Build history of the part. All positions in model axes, mm. Face numbers are marked on the shaded views. Give positions to 0.01 mm unless a question says otherwise; leave off trailing zeros. Order: outer loops, then holes, each group sorted by start corner. A loop starts at its lowest first (then second) coordinate and runs counter-clockwise, first axis right, second up. Notation, with made-up numbers: (-30.75, -37) - (18.25, -37) arc R13 ccw to (18.25, -32) - close; hole circle Ø3 at (71.5, -24.75). An arc over 180 degrees is marked (long way). Use a Markdown table: item, result.
from build123d import *

# Parameters (mm, degrees)
SKETCH1_R           = 2.5
BOSS_EXTRUDE1_DEPTH = 20
CHAMFER1_SIZE       = 0.1
CHAMFER1_SIZE2      = 0.235585237
CUT_EXTRUDE1_DEPTH  = 0.5
FILLET1_R           = 0.05


with BuildPart() as part:
    # Sketch1 → Boss-Extrude1 (new body)
    with BuildSketch(Plane(origin=(0, 0, 0), x_dir=(1, 0, 0), z_dir=(0, 1, 0))):
        with Locations(Location((0, 0, 0), (0, 0, 270))):
            Circle(SKETCH1_R)
    extrude(amount=BOSS_EXTRUDE1_DEPTH)

    # Chamfer1
    chamfer1_edges = [part.edges().sort_by_distance(p)[0] for p in [
        (0, 20, -2.5),
    ]]
    chamfer1_side = [part.faces().sort_by_distance(p)[0] for p in [
        (0, 10, -2.5),
    ]]
    chamfer(chamfer1_edges, length=CHAMFER1_SIZE, length2=CHAMFER1_SIZE2, reference=chamfer1_side[0])

    # Sketch2 → Cut-Extrude1 (cut)
    with BuildSketch(Plane(origin=(0, 20, 0), x_dir=(1, 0, 0), z_dir=(0, 1, 0))):
        Polygon((0.5, 0.5), (0.5, 1.5), (-0.5, 1.5), (-0.5, 0.5), (-1.5, 0.5), (-1.5, -0.5), (-0.5, -0.5), (-0.5, -1.5), (0.5, -1.5), (0.5, -0.5), (1.5, -0.5), (1.5, 0.5), align=None)
    extrude(amount=-CUT_EXTRUDE1_DEPTH, mode=Mode.SUBTRACT)

    # Fillet1
    fillet1_edges = [part.edges().sort_by_distance(p)[0] for p in [
        (-0.5, 19.5, -1),
        (0, 19.5, -1.5),
        (0.5, 19.5, -1),
        (1, 19.5, -0.5),
        (1.5, 19.5, 0),
        (1, 19.5, 0.5),
        (0.5, 19.5, 1),
        (0, 19.5, 1.5),
        (-0.5, 19.5, 1),
        (-1, 19.5, 0.5),
        (-1.5, 19.5, 0),
        (-1, 19.5, -0.5),
        (-0.5, 20, -1),
        (-1, 20, -0.5),
        (-1.5, 20, 0),
        (-1, 20, 0.5),
        (-0.5, 20, 1),
        (0, 20, 1.5),
        (0.5, 20, 1),
        (1, 20, 0.5),
        (1.5, 20, 0),
        (1, 20, -0.5),
        (0.5, 20, -1),
        (0, 20, -1.5),
    ]]
    fillet(fillet1_edges, radius=FILLET1_R)


solid = part.part
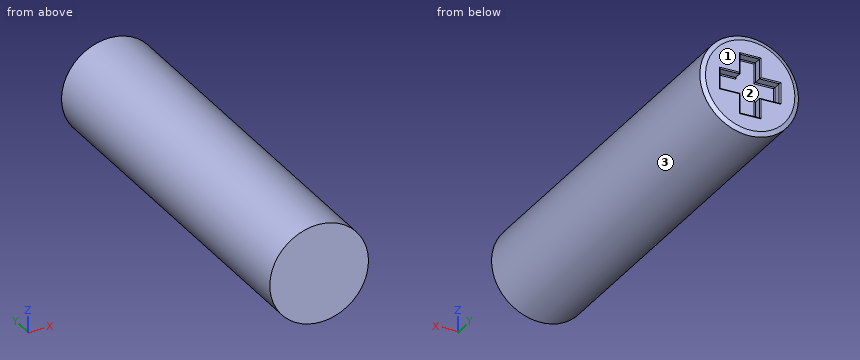
1) Pin check, flat tip, straight feed: P1, Ø1, axis at x = 0.5, y = 4, coming from the -Z side. Stop position of the tip, or through.
Computed:
| item | result |
|---|---|
| P1 | stops at z = -2.5 |
2) Slice it at C-C (y = 4.5). Write the cut outline in (x, z), and give its area (3 significant figures).
Computed:
| item | result |
|---|---|
| outline | circle Ø5 at (0, 0) |
| area | 19.6 mm² |
3) Wall check: line 1 (Y direction, x = -0.4, z = 1.15); line 2 (Y direction, x = -2.25, z = 0.3); line 3 (X direction, y = 19, z = -0.1). Give the ranges that are in metal, low to high. Write a range as from..to.
Computed:
| item | result |
|---|---|
| line 1 | y = 0..19.5 |
| line 2 | y = 0..20 |
| line 3 | x = -2.5..2.5 |
4) Slice it at B-B (z = 0). Write the cut outline in (x, y).
Computed:
| item | result |
|---|---|
| outline | (-2.5, 0) - (2.5, 0) - (2.5, 19.9) - (2.26, 20) - (1.55, 20) arc R0.05 ccw to (1.5, 19.95) - (1.5, 19.55) arc R0.05 cw to (1.45, 19.5) - (-1.45, 19.5) arc R0.05 cw to (-1.5, 19.55) - (-1.5, 19.95) arc R0.05 ccw to (-1.55, 20) - (-2.26, 20) - (-2.5, 19.9) - close |
5) Slice it at A-A (x = 0). Write the cut outline in (y, z), and give its area (3 significant figures).
Computed:
| item | result |
|---|---|
| outline | (0, -2.5) - (19.9, -2.5) - (20, -2.26) - (20, -1.55) arc R0.05 ccw to (19.95, -1.5) - (19.55, -1.5) arc R0.05 cw to (19.5, -1.45) - (19.5, 1.45) arc R0.05 cw to (19.55, 1.5) - (19.95, 1.5) arc R0.05 ccw to (20, 1.55) - (20, 2.26) - (19.9, 2.5) - (0, 2.5) - close |
| area | 98.5 mm² |
6) Two-plate mould, pull along X, no slides. Class the marked faces 1, 2 and 3: +X half, -X half, draft (parallel to the pull), parting line (faces both ways), or undercut.
Computed:
| item | result |
|---|---|
| face 1 | draft |
| face 2 | undercut |
| face 3 | parting line |
